Part model, mm, in its own coordinate system. Face numbers are marked on the shaded views. A direction names the side the tool comes from. Round coordinates to 2 decimals unless told otherwise and drop trailing zeros. Write each loop counter-clockwise with the first axis right and the second up, starting at its lowest first coordinate (ties: lowest second). Pieces come first, ordered by that corner, then holes. Notation, with made-up numbers: M 3.5,-29.5 L 30.5,-29.5 A28 ccw 30.5,-4.5 Z; hole C -23.75,-25 d4. An arc over 180 degrees is marked long. Answer as a JSON object with one key per item and string values. Group by question number.
1. Band-saw the part on C-C, the plane z = -34. Write the cut outline in (x, y), plus the area to 3 significant figures.
2. Drop flat-ended pins along their axis: pin 1 (2 mm diameter, centred on x = 5.5, z = 16, fed in from -Y); pin 2 (4 mm diameter, centred on x = -53, z = 1, fed in from -Y); pin 3 (8 mm diameter, centred on x = 20.5, z = 18, fed in from +Y). Give the stop position or say it passes through.
3. Band-saw the part on D-D, the plane y = 14.5. Write the cut outline in (x, z).
4. Band-saw the part on B-B, the plane x = -14.5. Write the cut outline in (y, z).
5. Two-plate mould, pull along Z, no slides. Class the marked faces 1, 2 and 3: +Z half, -Z half, draft (parallel to the pull), parting line (faces both ways), or undercut.
6. Band-saw the part on A-A, the plane y = 81. Write the cut outline in (x, z).
7. Which spindle directions (+Z, -Z, +X, -X, +Y, -Y) get a long thin tool onto all of the face, cutting with end or side? Do the marked faces 4, 5 and 6. Say none if no direction does.
8. Drill centre lines: line 1 (X direction, y = 19.5, z = -1); line 2 (Z direction, x = 5.5, y = 35.5); line 3 (Y direction, x = -22, z = 11). Where is each one in solid material? Low to high. Write a range as from..to.
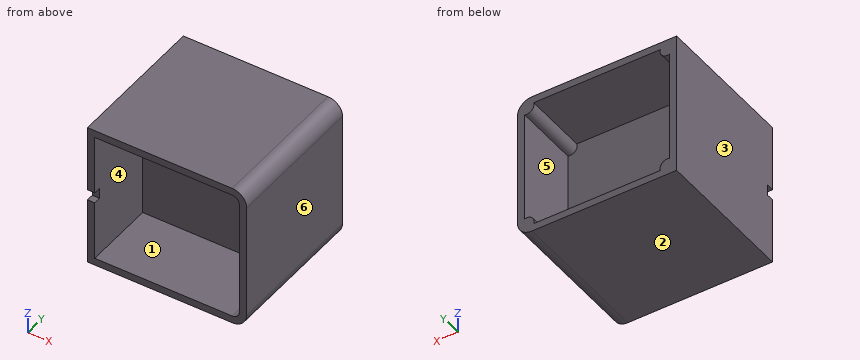
from build123d import *

# Parameters (mm, degrees)
BOSS_EXTRUDE1_DEPTH = 100
CUT_EXTRUDE1_DEPTH  = 50
CUT_EXTRUDE2_START  = -45
CUT_EXTRUDE2_DEPTH  = 45
SKETCH4_R           = 5
BOSS_EXTRUDE2_DEPTH = 45
SKETCH5_W           = 7.5
SKETCH5_H           = 5
CUT_EXTRUDE4_DEPTH  = 5


with BuildPart() as part:
    # Sketch1 → Boss-Extrude1 (new body)
    with BuildSketch(Plane(origin=(0, 0, 0), x_dir=(1, 0, 0), z_dir=(0, 1, 0))):
        with BuildLine():
            Line((-55, -50), (45, -50))
            ThreePointArc((45, -50), (52.071067812, -47.071067812), (55, -40))
            Line((55, -40), (55, 40))
            ThreePointArc((55, 40), (52.071067812, 47.071067812), (45, 50))
            Line((45, 50), (-55, 50))
            Line((-55, 50), (-55, -50))
        make_face()
    extrude(amount=BOSS_EXTRUDE1_DEPTH)

    # Sketch2 → Cut-Extrude1 (cut)
    with BuildSketch(Plane.XZ):
        with BuildLine():
            Line((-50, 45), (-50, -45))
            Line((-50, -45), (45, -45))
            ThreePointArc((45, -45), (48.535533906, -43.535533906), (50, -40))
            Line((50, -40), (50, 40))
            ThreePointArc((50, 40), (48.535533906, 43.535533906), (45, 45))
            Line((45, 45), (-50, 45))
        make_face()
    extrude(amount=-CUT_EXTRUDE1_DEPTH, mode=Mode.SUBTRACT)

    # Sketch3 → Cut-Extrude2 (cut)
    with BuildSketch(Plane(origin=(0, 100, 0), x_dir=(1, 0, 0), z_dir=(0, 1, 0)).offset(CUT_EXTRUDE2_START)):
        with BuildLine():
            Line((-50, 45), (-50, -45))
            Line((-50, -45), (45, -45))
            ThreePointArc((45, -45), (48.535533906, -43.535533906), (50, -40))
            Line((50, -40), (50, 40))
            ThreePointArc((50, 40), (48.535533906, 43.535533906), (45, 45))
            Line((45, 45), (-50, 45))
        make_face()
    extrude(amount=CUT_EXTRUDE2_DEPTH, mode=Mode.SUBTRACT)

    # Sketch4 → Boss-Extrude2 (add)
    with BuildSketch(Plane(origin=(0, 100, 0), x_dir=(1, 0, 0), z_dir=(0, 1, 0))):
        with Locations((48.535533906, -43.535533906)):
            Circle(SKETCH4_R)
        with Locations((48.535533906, 43.535533906)):
            Circle(SKETCH4_R)
        with Locations((-48.535533906, -43.535533906)):
            Circle(SKETCH4_R)
        with Locations((-48.535533906, 43.535533906)):
            Circle(SKETCH4_R)
    extrude(amount=-BOSS_EXTRUDE2_DEPTH)

    # Sketch5 → Cut-Extrude4 (cut)
    with BuildSketch(Plane.ZY.offset(55)):
        with Locations((0, 2.5)):
            Rectangle(SKETCH5_W, SKETCH5_H)
    extrude(amount=-CUT_EXTRUDE4_DEPTH, mode=Mode.SUBTRACT)


solid = part.part
Worked answers:
{
 "1": {"outline": "M -55,0 L -50,0 L -50,50 L 50,50 L 50,0 L 55,0 L 55,100 L 50,100 L 50,55 L -50,55 L -50,100 L -55,100 Z", "area": "1,500 mm^2"},
 "2": {"pin 1": "stops at y = 50", "pin 2": "stops at y = 5", "pin 3": "stops at y = 55"},
 "3": {"outline": "M -55,-50 L 45,-50 A10 ccw 55,-40 L 55,40 A10 ccw 45,50 L -55,50 Z; hole M -50,-45 L 45,-45 A5 ccw 50,-40 L 50,40 A5 ccw 45,45 L -50,45 Z"},
 "4": {"outline": "M 0,-50 L 100,-50 L 100,-45 L 55,-45 L 55,45 L 100,45 L 100,50 L 0,50 L 0,45 L 50,45 L 50,-45 L 0,-45 Z"},
 "5": {"face 1": "undercut", "face 2": "-Z half", "face 3": "draft"},
 "6": {"outline": "M -55,-50 L 45,-50 A10 ccw 55,-40 L 55,40 A10 ccw 45,50 L -55,50 Z; hole M -50,-38.75 A5 cw -43.75,-45 L 43.75,-45 A5 cw 50,-38.75 L 50,38.75 A5 cw 43.75,45 L -43.75,45 A5 cw -50,38.75 Z"},
 "7": {"face 4": "-Y", "face 5": "+Y", "face 6": "+Z, -Z, +X, +Y, -Y"},
 "8": {"line 1": "x = -55..-50, 50..55", "line 2": "z = -50..-45, 45..50", "line 3": "y = 50..55"}
}
